Build history of the part. All positions in model axes, mm. A direction names the side the tool comes from. Coordinates: 2 decimals unless noted, no trailing zeros. Write each loop counter-clockwise with the first axis right and the second up, starting at its lowest first coordinate (ties: lowest second). Pieces come first, ordered by that corner, then holes.
from build123d import *

# Parameters (mm, degrees)
F1_DEPTH = 10.16
F3_DEPTH = 7.62
F5_DEPTH = 2.54


with BuildPart() as f1:
    # F0 (on Top) → F1 (new body)
    with BuildSketch(Plane.XY):
        Polygon((-101.6, 0), (0, 0), (0, 10.16), (-200.0793895292, 10.16), (-200.0793895292, 0), (-123.8793895292, 0), (-56.4698083562, -24.5350810513), (-53.8636148641, -17.3746232809), align=None)
    extrude(amount=F1_DEPTH)

    # F2 (on face) → F3 (cut)
    with BuildSketch(Plane.XY.offset(10.16)):
        Polygon((-54.2979804461, -18.5680329093), (-115.9915508729, 3.8865903716), (-115.5571852908, 5.08), (-105.0892963227, 1.27), (0, 1.27), (0, 8.89), (-200.0793895292, 8.89), (-200.0793895292, 1.27), (-123.6554542637, 1.27), (-56.0354427742, -23.3416714229), align=None)
    extrude(amount=-F3_DEPTH, mode=Mode.SUBTRACT)

    # F4 (on face) → F5 (join)
    with BuildSketch(Plane.XY.offset(10.16)):
        Polygon((-101.6, 0), (0, 0), (0, 10.16), (-200.0793895292, 10.16), (-200.0793895292, 0), (-123.8793895292, 0), (-56.4698083562, -24.5350810513), (-53.8636148641, -17.3746232809), align=None)
    extrude(amount=F5_DEPTH)


solid = f1.part
(1) Slice it at B-B, the plane x = -73. List the corners of the cut face in (y, z).
(2) Slice it at D-D, the plane y = -11.5. List the corners of the cut face in (x, z), and give its area (3 significant figures).
(3) Slice it at C-C, the plane x = -154. List the corners of the cut face in (y, z).
(4) Two-plate mould, pull along Y, no slides. Class faces 5 (the flat face through (-90.646, -12.096, 6.261)), 6 (the flat face through (-99, 10.16, 6)), 7 (the flat face through (-110.397, 3.202, 6.403)): pulls with the +Y half, pulls with the -Y half, needs draft (parallel to the pull), parting line crosses it, or undercut.
(5) 3-axis set-ups, long thin cutter, end or side, ignore diameter. For faces 1 (the flat face through (-90.319, -10.864, 6.403)), 2 (the flat face through (-99, 8.89, 6)), 3 (the flat face through (-77.4, -8.81, 6.26)), 4 (the flat face through (-163, 0, 6)): which of +Z, -Z, +X, -X, +Y, -Y reach the whole face in a straight line?
(6) Slice it at A-A, the plane z = 8.25. List the corners of the cut face in (x, y), and give its area (3 significant figures).
(7) Probe L1, parallel to Y at x = -160, z = 8.5; L2, parallel to Z at x = -122, y = 4.5; L3, parallel to Y at x = -188, z = 0.5. List the from-to ranges inside material, lowest first.
(8) Flat gauge pin, fed straight in: P1, Ø5, axis at x = -46, z = 10.5, coming from the -Y side. Where does the tip first touch, or does it go through?
Results:
1. outline: (-18.52, 0) - (-10.41, 0) - (-10.41, 12.7) - (-18.52, 12.7) - close; (0, 0) - (10.16, 0) - (10.16, 12.7) - (0, 12.7) - close; hole (-17.17, 2.54) - (-11.76, 2.54) - (-11.76, 10.16) - (-17.17, 10.16) - close; hole (1.27, 2.54) - (8.89, 2.54) - (8.89, 10.16) - (1.27, 10.16) - close
2. outline: (-92.28, 0) - (-70, 0) - (-70, 12.7) - (-92.28, 12.7) - close; hole (-88.57, 2.54) - (-73.72, 2.54) - (-73.72, 10.16) - (-88.57, 10.16) - close
2. area: 170 mm2
3. outline: (0, 0) - (10.16, 0) - (10.16, 12.7) - (0, 12.7) - close; hole (1.27, 2.54) - (8.89, 2.54) - (8.89, 10.16) - (1.27, 10.16) - close
4. face 5: pulls with the -Y half
4. face 6: pulls with the +Y half
4. face 7: undercut
5. face 1: none
5. face 2: +X, -X
5. face 3: +Z, -Z, +X
5. face 4: +Z, -Z, -X, -Y
6. outline: (-200.08, 0) - (-123.88, 0) - (-56.47, -24.54) - (-56.04, -23.34) - (-123.66, 1.27) - (-200.08, 1.27) - close; (-200.08, 8.89) - (0, 8.89) - (0, 10.16) - (-200.08, 10.16) - close; (-115.99, 3.89) - (-54.3, -18.57) - (-53.86, -17.37) - (-101.6, 0) - (0, 0) - (0, 1.27) - (-105.09, 1.27) - (-115.56, 5.08) - close
6. area: 657 mm2
7. L1: y = 0 to 1.27, 8.89 to 10.16
7. L2: z = 0 to 2.54, 10.16 to 12.7
7. L3: y = 0 to 10.16
8. P1: stops at y = 0
